Answer from the drawing. Dimensions are ordinates in mm from the lowest x, y and z of the part. A direction names the side the tool comes from. Round coordinates to 2 decimals unless told otherwise and drop trailing zeros. Loops run counter-clockwise (first coordinate to the right, second up) from the corner with the lowest first, then second, coordinate; pieces in that order, holes last. Notation, with made-up numbers: (-13, -13.5) - (16, -13.5) arc R10 cw to (16, -0.5) - close; hole circle Ø6 at (68, 38). An arc over 180 degrees is marked (long way). Write item = value, one per line. Start each with the question number.
1) Section B-B, the plane y = 108 is taken. Determine the outline of the cut face in (x, z), and give its area (3 significant figures).
2) For a pull along X with two mould halves and no side action, classify the marked faces 3, 4, 5 and 6 as released by +X, released by -X, zero draft, split by the parting line, or undercut.
3) A tool of negligible diameter and unlimited length cuts with its end or side. For the marked faces 1 and 2, from which of +Z, -Z, +X, -X, +Y, -Y can it reach the whole face along a straight path? Write none if from no direction.
4) Section A-A, the plane x = 65.5 is taken. Determine the outline of the cut face in (y, z), and give its area (3 significant figures).
5) Given pin 1 Ø4 at (x, z) = (10.5, 12) entering from +Y; pin 2 Ø3 at (x, z) = (46, 28.5) entering from +Y; pin 3 Ø2 at (y, z) = (55.59, 41.09) entering from -X; pin 4 Ø1.9 at (x, z) = (53, 10) entering from +Y, each flat-ended and moving along its own axis, determine where each tip first touches the part or whether it passes through.
6) Straight lines are drawn through the part: line 1 along Y through (x, z) = (89, 22) (1 decimal); line 2 along X through (y, z) = (95.5, 5); line 3 along X through (y, z) = (5, 10). For each, find the intervals that lie inside material, in ascending order.
7) Section C-C, the plane z = 22.5 is taken. Give the number of separate pieces and of enclosed holes in the cut face, and give its area (3 significant figures).
8) Section D-D, the plane y = 84 is taken. Determine the outline of the cut face in (x, z), and give its area (3 significant figures).
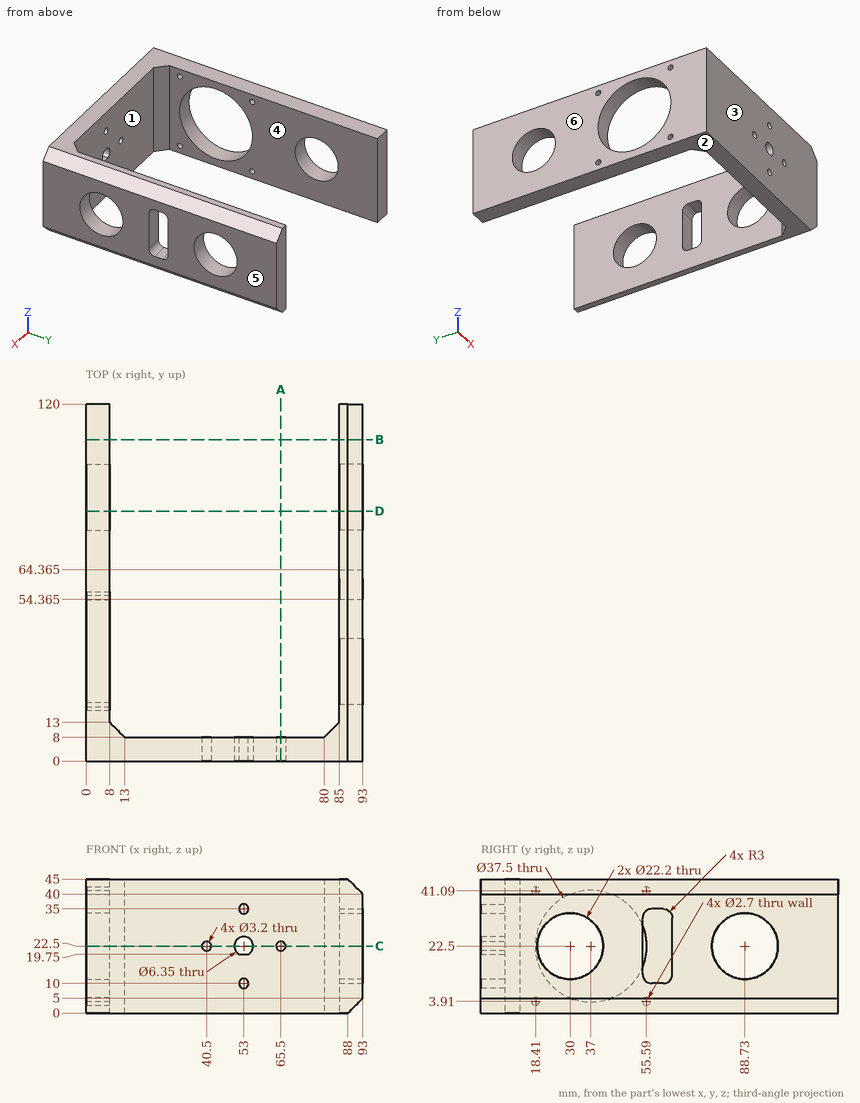
Geometry check:
q1.outline = (0, 0) - (8, 0) - (8, 45) - (0, 45) - close; (85, 0) - (88, 0) - (93, 5) - (93, 40) - (88, 45) - (85, 45) - close
q1.area = 695 mm2
q2.face_3 = zero draft
q2.face_4 = undercut
q2.face_5 = released by +X
q2.face_6 = released by -X
q3.face_1 = +Z, -Z, +Y
q3.face_2 = -Z, +X, -X, +Y, -Y
q4.outline = (0, 0) - (8, 0) - (8, 20.9) - (0, 20.9) - close; (0, 24.1) - (8, 24.1) - (8, 45) - (0, 45) - close
q4.area = 334 mm2
q5.pin_1 = 12.5
q5.pin_2 = 8
q5.pin_3 = 85
q5.pin_4 = through
q6.line_1 = 0 to 18.9, 41.1 to 54.4, 64.4 to 77.6, 99.8 to 120
q6.line_2 = 0 to 8, 85 to 93
q6.line_3 = 0 to 51.4, 54.6 to 93
q7.separate_pieces = 9
q7.enclosed_holes = 0
q7.area = 1,550 mm2
q8.outline = (0, 0) - (8, 0) - (8, 12.46) - (0, 12.46) - close; (0, 32.54) - (8, 32.54) - (8, 45) - (0, 45) - close; (85, 0) - (88, 0) - (93, 5) - (93, 12.46) - (85, 12.46) - close; (85, 32.54) - (93, 32.54) - (93, 40) - (88, 45) - (85, 45) - close
q8.area = 374 mm2
